Read the model definition and answer for the solid it produces. Units are mm, in the model's axes. Face numbers are marked on the shaded views. A direction names the side the tool comes from. Coordinates: 2 decimals unless noted, no trailing zeros. Loops run counter-clockwise (first coordinate to the right, second up) from the corner with the lowest first, then second, coordinate; pieces in that order, holes last. Notation, with made-up numbers: M 37,-39 L 54,-39 A24 ccw 54,-15 Z; hole C 0,76 d11. An arc over 180 degrees is marked long. Put each result on its own line as item: value.
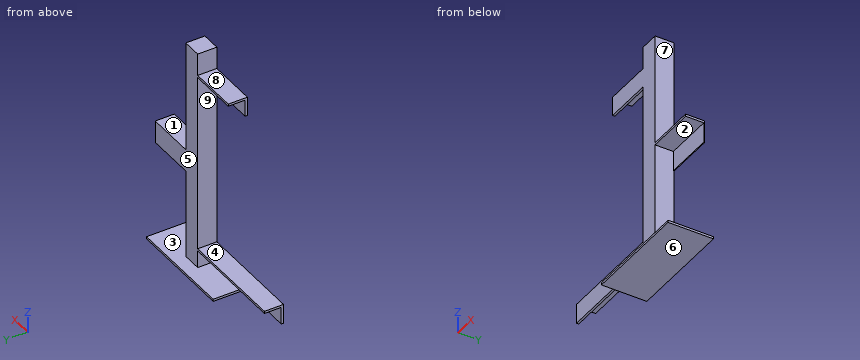
from build123d import *

# Parameters (mm, degrees)
SKETCH1_W             = 240
SKETCH1_H             = 101.6
BOSS_EXTRUDE1_DEPTH   = 5
SKETCH2_W             = 42.790852113
SKETCH2_H             = 42.790852114
BOSS_EXTRUDE2_DEPTH   = 500
BOSS_EXTRUDE3_DEPTH   = 110
BOSS_EXTRUDE4_DEPTH   = 110
BOSS_EXTRUDE4_2_DEPTH = 110
BOSS_EXTRUDE5_START   = 110
BOSS_EXTRUDE5_DEPTH   = 130


# Read off the part's stored shape, not the designer's step: Boss-Extrude3
with BuildPart() as part:
    # Sketch1 → Boss-Extrude1 (new body)
    with BuildSketch(Plane.XY.offset(40212.600196068)):
        with Locations((-22830.561141865, -1672.538517707)):
            Rectangle(SKETCH1_W, SKETCH1_H)
    extrude(amount=BOSS_EXTRUDE1_DEPTH)


with BuildPart() as body_2:
    # Sketch2 → Boss-Extrude2 (new body)
    with BuildSketch(Plane.XY.offset(40217.600196068)):
        with Locations((-22825.956567922, -1672.642858756)):
            Rectangle(SKETCH2_W, SKETCH2_H)
    extrude(amount=BOSS_EXTRUDE2_DEPTH)


with BuildPart() as body_3:
    # Boss-Extrude3 outline → Boss-Extrude3 (new body)
    with BuildSketch(Plane(origin=(-22804.561141865, 0, 0), x_dir=(0, 0, -1), z_dir=(1, 0, 0))):
        Polygon((-40467.600196068, -1694.038284813), (-40462.600196068, -1694.038284813), (-40462.600196068, -1653.231371608), (-40417.600196068, -1653.231371608), (-40417.600196068, -1651.247432699), (-40467.600196068, -1651.247432699), align=None)
    extrude(amount=BOSS_EXTRUDE3_DEPTH)


with BuildPart() as body_4:
    # Sketch4 → Boss-Extrude4 (new body)
    with BuildSketch(Plane.ZY.offset(22847.351993978)):
        Polygon((40667.600196068, -1651.247432699), (40662.600196068, -1651.247432699), (40662.600196068, -1689.038284813), (40624.809343955, -1689.038284813), (40624.809343955, -1694.038284813), (40667.600196068, -1694.038284813), align=None)
    extrude(amount=BOSS_EXTRUDE4_DEPTH)


with BuildPart() as body_5:
    # Sketch4 → Boss-Extrude4 2 (new body)
    with BuildSketch(Plane.ZY.offset(22847.351993978)):
        Polygon((40261.600196068, -1651.247432699), (40256.600196068, -1651.247432699), (40256.600196068, -1689.038284813), (40217.600196068, -1689.038284813), (40217.600196068, -1694.038284813), (40261.600196068, -1694.038284813), align=None)
    extrude(amount=BOSS_EXTRUDE4_2_DEPTH)

    # Sketch4<3> → Boss-Extrude5 (add)
    with BuildSketch(Plane.ZY.offset(22847.351993978).offset(BOSS_EXTRUDE5_START)):
        Polygon((40261.600196068, -1694.038284813), (40261.600196068, -1651.247432699), (40256.600196068, -1651.247432699), (40256.600196068, -1689.038284813), (40217.600196068, -1689.038284813), (40217.600196068, -1694.038284813), align=None)
    extrude(amount=BOSS_EXTRUDE5_DEPTH)


with BuildPart() as body_2_1:
    add(body_2.part)

    # Combine1: union body 3, body 4, body 5, part
    add(body_3.part)
    add(body_4.part)
    add(body_5.part)
    add(part.part)


solid = body_2_1.part
1) Which of the six approach directions +Z, -Z, +X, -X, +Y, -Y give full straight-line access (tool end or side, diameter ignored) to the marked faces 1, 2, 3, 4 and 5?
Answer list:
face 1: +Z, +X, +Y, -Y
face 2: +X, -Y
face 3: none
face 4: -X, +Y, -Y
face 5: +Z, +X, -X, +Y
2) Determine the mould class of the marked faces 6, 7, 8 and 9 for opening direction Z: released by +Z, released by -Z, zero draft, split by the parting line, or undercut.
Answer list:
face 6: released by -Z
face 7: zero draft
face 8: released by +Z
face 9: undercut
3) Find section A-A, the plane x = -22919.5. Write down the section's boundary in (y, z), plus the area to 3 significant figures.
Answer list:
outline: M -1723.34,40212.6 L -1621.74,40212.6 L -1621.74,40217.6 L -1689.04,40217.6 L -1689.04,40256.6 L -1651.25,40256.6 L -1651.25,40261.6 L -1694.04,40261.6 L -1694.04,40217.6 L -1723.34,40217.6 Z; M -1694.04,40624.81 L -1689.04,40624.81 L -1689.04,40662.6 L -1651.25,40662.6 L -1651.25,40667.6 L -1694.04,40667.6 Z
area: 1,320 mm^2
4) Find section C-C, the plane y = -1664.5. Write down the section's boundary in (x, z).
Answer list:
outline: M -23087.35,40256.6 L -22847.35,40256.6 L -22847.35,40217.6 L -22950.56,40217.6 L -22950.56,40212.6 L -22710.56,40212.6 L -22710.56,40217.6 L -22804.56,40217.6 L -22804.56,40462.6 L -22694.56,40462.6 L -22694.56,40467.6 L -22804.56,40467.6 L -22804.56,40717.6 L -22847.35,40717.6 L -22847.35,40667.6 L -22957.35,40667.6 L -22957.35,40662.6 L -22847.35,40662.6 L -22847.35,40261.6 L -23087.35,40261.6 Z
5) Straight lines are drawn through the part: line 1 (Z direction, x = -22913, y = -1654); line 2 (Z direction, x = -22713, y = -1688); line 3 (Z direction, x = -22762, y = -1700). For each, find the intervals that lie inside material, in ascending order. Write a range as [from, to].
Answer list:
line 1: z = [40212.6, 40217.6], [40256.6, 40261.6], [40662.6, 40667.6]
line 2: z = [40212.6, 40217.6], [40462.6, 40467.6]
line 3: z = [40212.6, 40217.6]
6) Find section B-B, the plane x = -22756. Write down the section's boundary in (y, z).
Answer list:
outline: M -1723.34,40212.6 L -1621.74,40212.6 L -1621.74,40217.6 L -1723.34,40217.6 Z; M -1694.04,40462.6 L -1653.23,40462.6 L -1653.23,40417.6 L -1651.25,40417.6 L -1651.25,40467.6 L -1694.04,40467.6 Z
7) Find section D-D, the plane z = 40454.5. Write down the section's boundary in (x, y), plus the area to 3 significant figures.
Answer list:
outline: M -22847.35,-1694.04 L -22804.56,-1694.04 L -22804.56,-1653.23 L -22694.56,-1653.23 L -22694.56,-1651.25 L -22847.35,-1651.25 Z
area: 2,050 mm^2
8) Given pin 1 Ø5.5 at (y, z) = (-1674, 40215) entering from -X; pin 2 Ø21.5 at (y, z) = (-1665.5, 40304.5) entering from +X; pin 3 Ø6 at (x, y) = (-22790.5, -1654) entering from +Z, each flat-ended and moving along its own axis, determine where each tip first touches the part or whether it passes through.
Answer list:
pin 1: stops at x = -22950.56
pin 2: stops at x = -22804.56
pin 3: stops at z = 40467.6
